Autodesk Fusion 360 part; units mm, degrees
sketch "スケッチ1" plane through (0, 0, 0) normal (0, 1, 0) x (1, 0, 0)
  line L0 (84.9076, 0) -> (-96.0768, 0) construction
  line L1 (0, -64.1732) -> (0, 68.3912) construction
  line L2 (0, -50) -> (-50, -50)
  line L3 (-50, -50) -> (-50, 50)
  line L4 (0, 50) -> (-50, 50)
  circle A0 centre (0, 0) radius 25
  arc A1 (0, -50) -> (0, 50) centre (0, 0) ccw
  line L5 (0, -47) -> (-50, -47)
  line L6 (0, 47) -> (-50, 47)
  arc A2 (0, -47) -> (0, 47) centre (0, 0) ccw
  circle A3 centre (0, 0) radius 30
  line L7 (-50, -47) -> (-52, -47)
  line L8 (-52, -47) -> (-52, 47)
  line L9 (-52, 47) -> (-50, 47)
  line L10 (-50, 47) -> (-50, -47)
  line L11 (-31.5, 57.8245) -> (-31.5, -58.1462) construction
  line L12 (-37.5, -7.5) -> (-25, -7.5)
  line L13 (-25, 7.5) -> (-37.5, 7.5)
  line L14 (-37.5, 7.5) -> (-37.5, -7.5)
  line L15 (-25, -7.5) -> (-23.8485, -7.5)
  line L16 (-25, 7.5) -> (-23.8485, 7.5)
  line L17 (-32.1391, -10) -> (-28.2843, -10) construction
  line L18 (-32.1391, 10) -> (-28.2843, 10) construction
  circle A4 centre (-31.5, -10) radius 1.35
  circle A5 centre (-31.5, 10) radius 1.35
  line L19 (-52, -27) -> (-50, -27.0394)
  line L20 (-52, 27) -> (-50, 27)
  dimension "d1" = 100
  dimension "d2" = 50
  dimension "d3" = 50
  dimension "d4" = 94
  dimension "d5" = 60
  dimension "d17" = 2
  dimension "d18" = 31.5
  dimension "d20" = 15
  dimension "d21" = 7.5
  dimension "d22" = 6
  dimension "d23" = 20
  dimension "d24" = 10
  dimension "d25" = 2.7
  dimension "d26" = 2.7
  dimension "d36" = 20
  dimension "d37" = 20
extrude "押し出し1" add sketch "スケッチ1" along normal blind 5 contours L2 L3 L4 A1 L5 L6 A2 | L3 L5 L6 A2 L10 | A3 L12 L13 L14 | A4 | A5
fillet "フィレット1" radius 2 3 edges at (-25, 5, 50) (50, 5, 0) (-25, 5, -50)
fillet "フィレット2" radius 2 1 edges at (-27.9698, 5, -10.8485)
extrude "押し出し3" add sketch "スケッチ1" against normal blind 2 contours L3 L7 L8 L10 L19 | L3 L5 L6 A2 L10 | L3 L8 L10 L19 L20 | L3 L8 L9 L10 L20 | A0 A3 L12 L13 L15 L16 | A0 A3 L12 L13 L15 L16 | A3 L12 L13 L14 | A4 | A5
extrude "押し出し7" add sketch "スケッチ1" along normal blind 2 contours A0 A3 L12 L13 L15 L16 | A0 A3 L12 L13 L15 L16
extrude "押し出し8" cut 1 faces at (-33.3333, 0, -49) along direction (0, 1, 0) blind 0.5
extrude "押し出し9" cut 1 faces at (-51.3333, 0, -15.6667) along direction (0, -1, 0) blind 0.5
extrude "押し出し4" cut sketch "スケッチ1" along normal blind 2.5 from surface at -2 contours A0 A3 L12 L13 L15 L16 | A3 L12 L13 L14 picked at (-17.5252, -22.1967)
extrude "押し出し5" add sketch "スケッチ1" along normal blind 3 from surface at -2 contours A4 | A5
extrude "押し出し6" cut sketch "スケッチ1" along normal blind 5 from surface at -2 contours L3 L7 L8 L10 L19 | L3 L8 L9 L10 L20 | A4 | A5
equation "d21 = d20 / 2"
equation "d24 = d23 / 2"
Design review of the part built by this model. Coordinates are the model's own, in mm. A direction names the side the tool comes from. Coordinates: 2 decimals unless noted, no trailing zeros. Write each loop counter-clockwise with the first axis right and the second up, starting at its lowest first coordinate (ties: lowest second). Pieces come first, ordered by that corner, then holes. Notation, with made-up numbers: (-22.75, 75) -> (15.25, 75) arc R19 cw to (15.25, 95) -> close; hole circle Ø8 at (-12.5, 52.25). An arc over 180 degrees is marked (long way). Write each question's results on one line, items separated by ' | '. Start each with the question number.
(1) For line 1 along X through (y, z) = (-1, 1); line 2 along X through (y, z) = (-0.4, 0); line 3 along Z through (x, y) = (-31.5, -0.45), list the stretches that pass through material, from the lowest coordinate up. Write a range as from..to.
(2) Clearance check with flat-ended pins moving along their axes: P1, Ø1.5, axis at y = -1, z = 22, coming from the +X side; P2, Ø3, axis at y = 1, z = -39.5, coming from the +X side; P3, Ø1.3, axis at x = -31, z = 10, coming from the -Y side; P4, Ø18, axis at x = -11.5, z = -4.5, coming from the +Y side. State where each tip first meets the part, or that it passes through.
(3) The part is to be moulded in two halves that separate along X. For faces 1 (the face through (-25, -1, 47)), 2 (the face through (49.988, 1.732, -1.099)), 3 (the face through (-26, -1, -7.5)), say which applies: pulls with the +X half, pulls with the -X half, needs draft (parallel to the pull), parting line crosses it, or undercut.
(4) Take a section at A-A on z = 0. Write out the cut boundary in (x, y).
(5) Tool access review of faces 4 (the face through (-25, 2, 50)), 5 (the face through (-33, 0.5, 0)), 6 (the face through (-29.97, 2.49, 1.32)), 7 (the face through (-25, -1, -47)), 8 (the face through (48, 0.5, 0)): name each direction out of +Z, -Z, +X, -X, +Y, -Y from which nothing blocks a thin tool from reaching the whole face with its end or side.
Results found:
1) line 1: x = -52..-37.5, -29.98..-24.98, 29.98..46.99 | line 2: x = -50..-37.5, -30..-25, 30..47 | line 3: z = -47..-11.35, -8.65..-7.5, 7.5..8.65, 11.35..47
2) P1: stops at x = 41.92 | P2: stops at x = 32.5 | P3: stops at y = 3 | P4: passes through
3) face 1: needs draft | face 2: pulls with the +X half | face 3: undercut
4) outline: (-52, -2) -> (-37.5, -2) -> (-37.5, 0.5) -> (-30, 0.5) -> (-30, -2) -> (-25, -2) -> (-25, 2) -> (-30, 2) -> (-30, 3) arc R2 ccw to (-32, 5) -> (-50, 5) -> (-50, -0.5) -> (-52, -0.5) -> close; (25, 0.5) -> (30, 0.5) -> (30, -2) -> (47, -2) -> (47, 0.5) -> (50, 0.5) -> (50, 3) arc R2 ccw to (48, 5) -> (32, 5) arc R2 ccw to (30, 3) -> (30, 2) -> (25, 2) -> close
5) face 4: +Z, +X, -X, +Y, -Y | face 5: -Y | face 6: +Y | face 7: -Z, +X, -X, -Y | face 8: +X, -Y
